Could you check a few things on this model? Use its own coordinates, in mm. A direction names the side the tool comes from. Give positions to 0.01 mm unless a question says otherwise; leave off trailing zeros. Loops run counter-clockwise (first coordinate to the right, second up) from the corner with the lowest first, then second, coordinate; pieces in that order, holes last. Notation, with made-up numbers: M 47,57 L 103,57 A12 ccw 103,72 Z; hole C -3,78.25 d6. An arc over 180 degrees is marked long. Answer in a Markdown table with one row per item. Add a question column.
1. Thinking about a two-plate mould opening in X: for faces 1 (the cylindrical face through (-2.75, -8.23, -12.4)), 2 (the flat face through (3, -6.35, 6)), which applies, released by +X, released by -X, zero draft, split by the parting line, or undercut?
2. I need wall thicknesses on line 1 along Y through (x, z) = (-5.75, 3); line 2 along Z through (x, y) = (11, -6.75); line 3 along Z through (x, y) = (-3.25, -0.25). Which ranges of each line are inside material? Lowest first, please. Write a range as from..to.
3. I'm going to push flat-ended pins straight in: pin 1 Ø3 at (x, z) = (0, -8.5) entering from +Y; pin 2 Ø3 at (y, z) = (3, 2) entering from -X. Where does each tip first touch, or does it pass through?
4. Which directions (+Z, -Z, +X, -X, +Y, -Y) give clear straight access to the entire face, cutting with the end or side of a thin tool? Please do faces 3 (the flat face through (0, -12.7, 0)), 4 (the cylindrical face through (-1.38, -0.09, -6.2)).
5. If we section it at B-B on z = 0: List the corners of the cut face in (x, y) for me.
6. If we section it at C-C on y = 4: List the corners of the cut face in (x, z) for me, then the cut area to 3 significant figures.
7. If we section it at D-D on y = -7.75: List the corners of the cut face in (x, z) for me.
8. If we section it at A-A on x = 0: List the corners of the cut face in (y, z) for me.
```python
from build123d import *

# Parameters (mm, degrees)
F0_R     = 6.35
F1_DEPTH = 6.35
F2_R     = 12.7
F3_DEPTH = 6.35
F4_R     = 2.54


with BuildPart() as f1:
    # F0 (on Front) → F1 (new body, symmetric)
    with BuildSketch(Plane.XZ):
        Circle(F0_R)
    extrude(amount=F1_DEPTH, both=True)

    # F2 (on face) → F3 (join)
    with BuildSketch(Plane.XZ.offset(6.35)):
        Circle(F2_R)
    extrude(amount=F3_DEPTH)

    # F4
    f4_edges = [f1.edges().sort_by_distance(p)[0] for p in [
        (-12.7, -12.7, 0),
    ]]
    fillet(f4_edges, radius=F4_R)


solid = f1.part
```
Results:
| question | item | result |
|---|---|---|
| 1 | face 1 | split by the parting line |
| 1 | face 2 | zero draft |
| 2 | line 1 | -12.7..-6.35 |
| 2 | line 2 | -6.35..6.35 |
| 2 | line 3 | -5.46..5.46 |
| 3 | pin 1 | y = -6.35 |
| 3 | pin 2 | x = -6.33 |
| 4 | face 3 | +Z, -Z, +X, -X, -Y |
| 4 | face 4 | +Y |
| 5 | outline | M -12.7,-10.16 A2.54 ccw -10.16,-12.7 L 10.16,-12.7 A2.54 ccw 12.7,-10.16 L 12.7,-6.35 L 6.35,-6.35 L 6.35,6.35 L -6.35,6.35 L -6.35,-6.35 L -12.7,-6.35 Z |
| 6 | outline | C 0,0 d12.7 |
| 6 | area | 127 mm2 |
| 7 | outline | C 0,0 d25.4 |
| 8 | outline | M -12.7,-10.16 A2.54 ccw -10.16,-12.7 L -6.35,-12.7 L -6.35,-6.35 L 6.35,-6.35 L 6.35,6.35 L -6.35,6.35 L -6.35,12.7 L -10.16,12.7 A2.54 ccw -12.7,10.16 Z |
